from build123d import *


with BuildPart() as part:
    # Sketch3 → Revolve1 (revolve)
    with BuildSketch(Plane.XY, mode=Mode.PRIVATE) as revolve1_sk:
        with BuildLine():
            Line((-14.647440478, 1.4), (-14.647440478, 15.08125))
            ThreePointArc((-14.647440478, 15.08125), (-13.150997434, 15.404541787), (-11.647440478, 15.69294401))
            Line((-11.647440478, 15.69294401), (-11.647440478, 3.4))
            Line((-11.647440478, 3.4), (-1.5, 3.4))
            Line((-1.5, 3.4), (-1.5, 16.71452719))
            ThreePointArc((-1.5, 16.71452719), (0, 16.731620181), (1.5, 16.71452719))
            Line((1.5, 16.71452719), (1.5, 3.4))
            Line((1.5, 3.4), (11.647440478, 3.4))
            Line((11.647440478, 3.4), (11.647440478, 15.69294401))
            ThreePointArc((11.647440478, 15.69294401), (13.150997434, 15.404541787), (14.647440478, 15.08125))
            Line((14.647440478, 15.08125), (14.647440478, 1.4))
            Line((14.647440478, 1.4), (-14.647440478, 1.4))
        make_face()
    revolve(revolve1_sk.sketch.rotate(Axis((23.642125672, 0, 0), (-1, 0, 0)), 90), axis=Axis((23.642125672, 0, 0), (-1, 0, 0)))

    # Sketch4 → Revolve2 (revolve)
    with BuildSketch(Plane.XY, mode=Mode.PRIVATE) as revolve2_sk:
        with BuildLine():
            Line((-14.647440478, 12.08125), (-14.647440478, 15.08125))
            ThreePointArc((-14.647440478, 15.08125), (0, 16.731620181), (14.647440478, 15.08125))
            Line((14.647440478, 15.08125), (14.647440478, 12.08125))
            ThreePointArc((14.647440478, 12.08125), (0, 13.731620181), (-14.647440478, 12.08125))
        make_face()
    revolve(revolve2_sk.sketch.rotate(Axis((23.642125672, 0, 0), (-1, 0, 0)), 270), axis=Axis((23.642125672, 0, 0), (-1, 0, 0)))


solid = part.part
Part model, mm, in its own coordinate system. A direction names the side the tool comes from. Coordinates: 2 decimals unless noted, no trailing zeros. Write each question's results on one line, items separated by ' | '. Start each with the question number.
Q1. Slice it at A-A on y = 0. Give the number of separate pieces and of enclosed holes in the cut face, and give its area (3 significant figures).
Q2. Which spindle directions (+Z, -Z, +X, -X, +Y, -Y) get a long thin tool onto all of the face, cutting with end or side? Do faces 1 (the flat face through (11.647, 3, 3)), 2 (the flat face through (-14.647, 3, 0)). Say none if no direction does.
Q3. Probe line 1 along X through (y, z) = (11, 5); line 2 along Y through (x, z) = (-2.25, 0); line 3 along Y through (x, z) = (5, -1.5). List the from-to ranges inside material, lowest first.
Q4. Two-plate mould, pull along Z, no slides. Class faces 3 (the flat face through (-1.5, 3, 3)), 4 (the flat face through (14.647, 3, 0)): +Z half, -Z half, draft (parallel to the pull), parting line (faces both ways), or undercut.
Q5. Drop flat-ended pins along their axis: pin 1 Ø6 at (x, y) = (3, -1) entering from +Z; pin 2 Ø1.5 at (x, z) = (4, 9.5) entering from +Y; pin 3 Ø2 at (x, y) = (5.5, -5) entering from -Z. Give the stop position or say it passes through.
Answer:
1) separate pieces: 2 | enclosed holes: 4 | area: 463 mm2
2) face 1: none | face 2: +Z, -Z, -X, +Y, -Y
3) line 1: x = -14.65 to -11.65, -1.5 to 1.5, 11.65 to 14.65 | line 2: y = -16.69 to -13.69, -3.4 to -1.4, 1.4 to 3.4, 13.69 to 16.69 | line 3: y = -16.47 to -13.46, -3.05 to 3.05, 13.46 to 16.47
4) face 3: undercut | face 4: draft
5) pin 1: stops at z = 16.73 | pin 2: stops at y = 14.12 | pin 3: stops at z = -16.02
